The drawing under review shows one solid part. Ordinate dimensions are in mm from its lowest x, y, z. A direction names the side the tool comes from. Give positions to 0.01 mm unless a question says otherwise; leave off trailing zeros. Order: outer loops, then holes, each group sorted by start corner. A loop starts at its lowest first (then second) coordinate and runs counter-clockwise, first axis right, second up. Notation, with made-up numbers: (63, -12) - (80, -12) arc R25 cw to (80, 17) - close; hole circle Ø2 at (45.5, 26.5). An arc over 180 degrees is marked (long way). Write item = value, one per line. Start each with the question number.
1. We need section A-A, the plane x = 29. Give the boundary of the cut face in (y, z), and give its area (3 significant figures).
2. Wall thickness on probe 1 along X at (y, z) = (10.1, 29); probe 2 along X at (y, z) = (12.5, 29); probe 3 along Y at (x, z) = (45, 35): over which ranges is each line inside the solid? List them lowest first.
3. We need section B-B, the plane z = 29. Give the boundary of the cut face in (x, y), and give its area (3 significant figures).
4. We need section C-C, the plane y = 3.25. Give the boundary of the cut face in (x, z), and give its area (3 significant figures).
5. Mouldability with a two-part tool opening along Z and no side actions: class the marked faces 1, 2, 3 and 4 as pulls with the +Z half, pulls with the -Z half, needs draft (parallel to the pull), parting line crosses it, or undercut.
6. For P1, Ø1.5, axis at x = 44, z = 48, coming from the +Y side; P2, Ø12, axis at x = 44.5, y = 17.5, coming from the +Z side; P3, Ø6.5, axis at x = 40.5, z = 48.92, coming from the -Y side, all flat-tipped, find the tip position at first contact; note any pin that passes through.
7. We need section D-D, the plane x = 40.5. Give the boundary of the cut face in (y, z), and give its area (3 significant figures).
8. Machinability: for the marked faces 5, 6 and 7, which of the approach directions +Z, -Z, +X, -X, +Y, -Y give a long, thin tool a straight path to every point of the face, cutting with its end or side? Answer none if there is none.
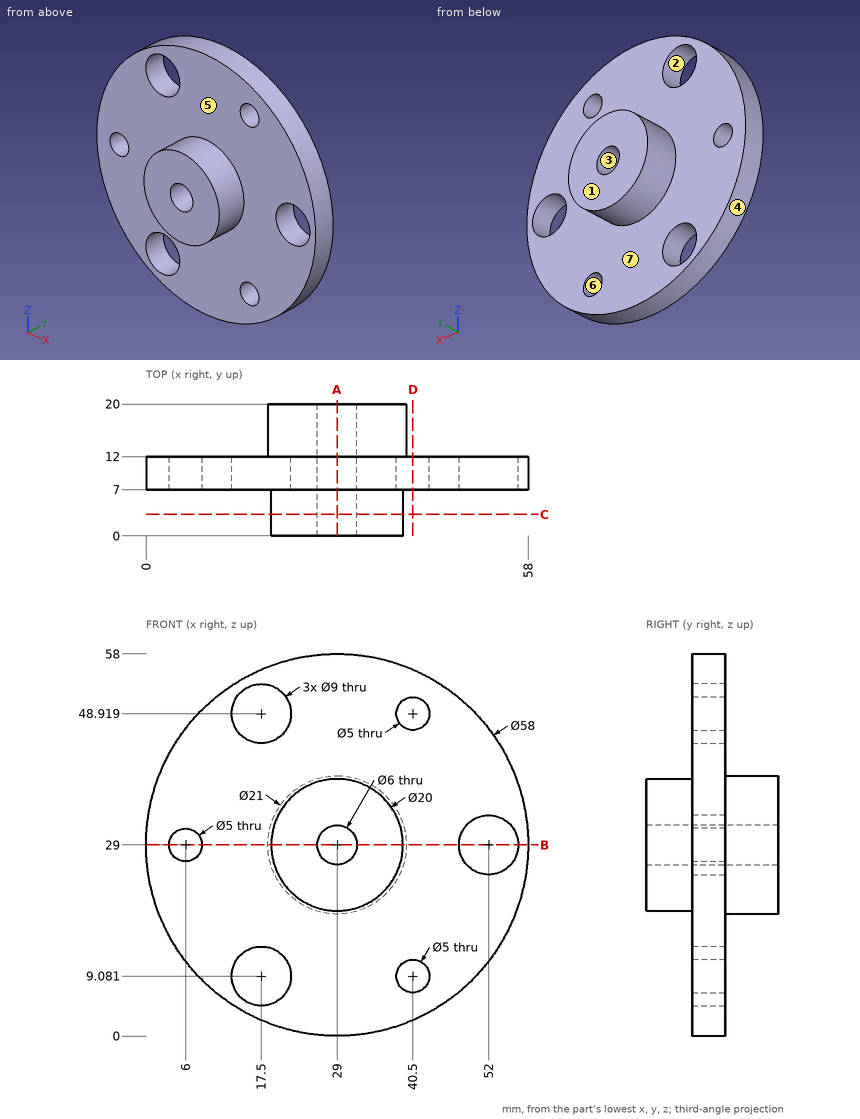
Model answer:
q1.outline = (0, 19) - (7, 19) - (7, 0) - (12, 0) - (12, 18.5) - (20, 18.5) - (20, 26) - (0, 26) - close; (0, 32) - (20, 32) - (20, 39.5) - (12, 39.5) - (12, 58) - (7, 58) - (7, 39) - (0, 39) - close
q1.area = 478 mm2
q2.probe_1 = 0 to 3.5, 8.5 to 26, 32 to 47.5, 56.5 to 58
q2.probe_2 = 18.5 to 26, 32 to 39.5
q2.probe_3 = 7 to 12
q3.outline = (0, 7) - (3.5, 7) - (3.5, 12) - (0, 12) - close; (8.5, 7) - (19, 7) - (19, 0) - (26, 0) - (26, 20) - (18.5, 20) - (18.5, 12) - (8.5, 12) - close; (32, 0) - (39, 0) - (39, 7) - (47.5, 7) - (47.5, 12) - (39.5, 12) - (39.5, 20) - (32, 20) - close; (56.5, 7) - (58, 7) - (58, 12) - (56.5, 12) - close
q3.area = 408 mm2
q4.outline = circle Ø20 at (29, 29); hole circle Ø6 at (29, 29)
q4.area = 286 mm2
q5.face_1 = needs draft
q5.face_2 = undercut
q5.face_3 = undercut
q5.face_4 = parting line crosses it
q6.P1 = 12
q6.P2 = 54.87
q6.P3 = 7
q7.outline = (7, 2.38) - (12, 2.38) - (12, 6.58) - (7, 6.58) - close; (7, 11.58) - (12, 11.58) - (12, 46.42) - (7, 46.42) - close; (7, 51.42) - (12, 51.42) - (12, 55.62) - (7, 55.62) - close
q7.area = 216 mm2
q8.face_5 = -Y
q8.face_6 = +Y, -Y
q8.face_7 = +Y
